Geometry check sheet. Reference: the model listing, model coordinates, mm. Face numbers are marked on the shaded views. A direction names the side the tool comes from. Give positions to 0.01 mm unless a question says otherwise; leave off trailing zeros. Write each loop counter-clockwise with the first axis right and the second up, starting at its lowest first coordinate (ties: lowest second). Pieces come first, ordered by that corner, then holes. Notation, with made-up numbers: (42.25, 1.5) -> (92.25, 1.5) arc R21 ccw to (92.25, 28.5) -> close; hole circle Ø2 at (-34, -2). An arc over 180 degrees is marked (long way). Write item = value, one per line. Start each with the question number.
1. Cross-section at D-D, the plane y = -2.5. Record the cut outline in (x, z).
2. Cross-section at C-C, the plane x = -18.5. Record the cut outline in (y, z), plus the area to 3 significant figures.
3. Cross-section at A-A, the plane y = 0. Record the cut outline in (x, z).
4. Thickness scan on line 1 along Y through (x, z) = (-0.5, 1); line 2 along X through (y, z) = (-2.5, 2.25); line 3 along X through (y, z) = (0.75, 2.75). Record the ranges inside material, lowest first.
5. Set-up check for the marked faces 1, 2, 3 and 4: record each of +Z, -Z, +X, -X, +Y, -Y from which the full face is reachable in a straight line by a thin tool's end or side.
6. Cross-section at B-B, the plane z = 0. Record the cut outline in (x, y).
7. Depth check by flat-ended pin: P1, Ø2, axis at x = -8.5, z = 0.5, coming from the -Y side; P2, Ø4, axis at x = 2, z = -2, coming from the -Y side; P3, Ø3, axis at x = -8.5, y = -2.5, coming from the -Z side. Enter the tip coordinate at first touch or a pass-through.
Autodesk Inventor part; units mm, degrees
ref_plane "YZ Plane" through (0, 0, 0) normal (1, 0, 0) x (0, 1, 0)
ref_plane "XZ Plane" through (0, 0, 0) normal (0, 1, 0) x (-1, 0, 0)
ref_plane "XY Plane" through (0, 0, 0) normal (0, 0, 1) x (1, 0, 0)
sketch "Sketch1" plane through (0, 0, 0) normal (1, 0, 0) x (0, 1, 0)
  circle A0 centre (0, 0) radius 3
  dimension "d0" = 6
extrude "Extrusion1" add sketch "Sketch1" along normal blind 17
sketch "Sketch2" plane through (17, 0, 0) normal (1, 0, 0) x (0, 0, -1)
  circle A0 centre (0, 0) radius 3.45
  dimension "d3" = 6.9
extrude "Extrusion2" add sketch "Sketch2" along normal blind 2.5
sketch "Sketch3" plane through (0, 0, 0) normal (-1, 0, 0) x (0, 0, 1)
  circle A0 centre (0, 0) radius 2.75
  dimension "d6" = 5.5
extrude "Extrusion3" add sketch "Sketch3" along normal blind 24
sketch "Sketch4" plane through (-24, 0, 0) normal (-1, 0, 0) x (0, 0, 1)
  line L0 (0, 0) -> (0, -1.85)
  line L1 (0, 0) -> (0, 1.85)
  line L2 (0, -1.85) -> (-3.7501, -1.85)
  line L3 (-3.7501, -1.85) -> (3.8768, -1.85)
  line L4 (3.8768, -1.85) -> (3.8768, 1.85)
  line L5 (3.8768, 1.85) -> (-3.7501, 1.85)
  line L6 (-3.7501, 1.85) -> (-3.7501, -1.85)
  line L7 (-7.0983, -8.0342) -> (8.0665, -8.0342)
  line L8 (8.0665, -8.0342) -> (8.0665, 8.0154)
  line L9 (8.0665, 8.0154) -> (-7.0983, 8.0154)
  line L10 (-7.0983, 8.0154) -> (-7.0983, -8.0342)
  dimension "d9" = 1.85
  dimension "d10" = 1.85
extrude "Extrusion4" cut sketch "Sketch4" against normal blind 24
properties part number "draaiarm voorwielen_3DPrint"
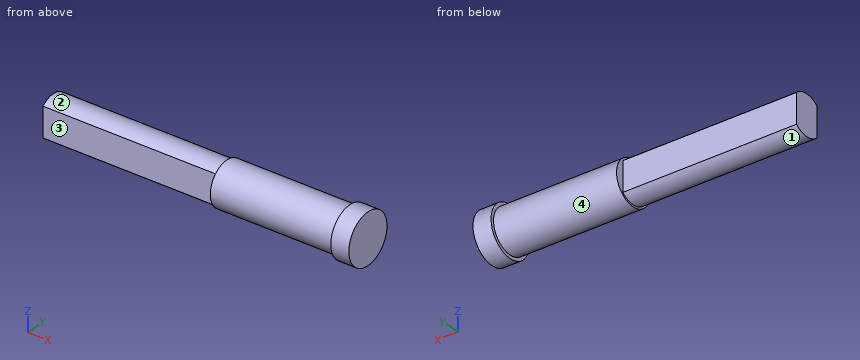
Answers:
q1.outline = (0, -1.66) -> (17, -1.66) -> (17, -2.38) -> (19.5, -2.38) -> (19.5, 2.38) -> (17, 2.38) -> (17, 1.66) -> (0, 1.66) -> close
q2.outline = (-1.85, -2.03) arc R2.75 ccw to (1.85, -2.03) -> (1.85, 2.03) arc R2.75 ccw to (-1.85, 2.03) -> close
q2.area = 18.7 mm^2
q3.outline = (-24, -2.75) -> (0, -2.75) -> (0, -3) -> (17, -3) -> (17, -3.45) -> (19.5, -3.45) -> (19.5, 3.45) -> (17, 3.45) -> (17, 3) -> (0, 3) -> (0, 2.75) -> (-24, 2.75) -> close
q4.line_1 = -1.85 to 1.85
q4.line_2 = 17 to 19.5
q4.line_3 = 0 to 19.5
q5.face_1 = -Z, -X
q5.face_2 = +Z, -X
q5.face_3 = +Z, -Z, -X, -Y
q5.face_4 = -X
q6.outline = (-24, -1.85) -> (0, -1.85) -> (0, -3) -> (17, -3) -> (17, -3.45) -> (19.5, -3.45) -> (19.5, 3.45) -> (17, 3.45) -> (17, 3) -> (0, 3) -> (0, 1.85) -> (-24, 1.85) -> close
q7.P1 = -1.85
q7.P2 = -3
q7.P3 = -2.56
